```python
from build123d import *

# Parameters (mm, degrees)
ESTRUSIONE1_DEPTH                                    = 200
M10_LAMATURA_PER_VITE_A_COPERTURA_CILIND_D           = 11
M10_LAMATURA_PER_VITE_A_COPERTURA_CILIND_CBORE_D     = 18
M10_LAMATURA_PER_VITE_A_COPERTURA_CILIND_CBORE_DEPTH = 10
RIPETIZIONE_A_L1_COUNT                               = 5
RIPETIZIONE_A_L1_PITCH                               = 42
RIPETIZIONE_A_L1_COUNT_DIR2                          = 2
RIPETIZIONE_A_L1_PITCH_DIR2                          = 160
SMUSSO1_SIZE                                         = 3
ESTRUSIONE2_DEPTH                                    = 223.712819568
M10_TAPPED_HOLE1_D                                   = 8.5
M10_TAPPED_HOLE1_DEPTH                               = 17.5
M10_TAPPED_HOLE1_TIP                                 = 2.553657631
SCHIZZO10_R                                          = 4
ESTRUSIONE3_DEPTH                                    = 12
ESTRUSIONE5_DEPTH                                    = 200
SMUSSO2_SIZE                                         = 2


with BuildPart() as part:
    # Schizzo1 → Estrusione1 (new body)
    with BuildSketch(Plane(origin=(0, 0, 0), x_dir=(1, 0, 0), z_dir=(0, 1, 0))):
        Polygon((0, -95), (0, 95), (-24, 95), (-24, 90), (-19, 90), (-19, 70), (-24, 70), (-24, -70), (-19, -70), (-19, -90), (-24, -90), (-24, -95), align=None)
    extrude(amount=ESTRUSIONE1_DEPTH)

    # M10 Lamatura per vite a copertura cilind (through all)
    with Locations(Plane(origin=(0, 0, 0), x_dir=(0, 0, -1), z_dir=(1, 0, 0))):
        with Locations((-80, 184)):
            m10_lamatura_per_vite_a_copertura_cilind = CounterBoreHole(M10_LAMATURA_PER_VITE_A_COPERTURA_CILIND_D / 2, M10_LAMATURA_PER_VITE_A_COPERTURA_CILIND_CBORE_D / 2, M10_LAMATURA_PER_VITE_A_COPERTURA_CILIND_CBORE_DEPTH)

    # Ripetizione a L1: M10 Lamatura per vite a copertura cilind 5 × 2
    with Locations(*[(0, -i * RIPETIZIONE_A_L1_PITCH, -j * RIPETIZIONE_A_L1_PITCH_DIR2) for i in range(RIPETIZIONE_A_L1_COUNT) for j in range(RIPETIZIONE_A_L1_COUNT_DIR2) if (i, j) != (0, 0)]):
        add(m10_lamatura_per_vite_a_copertura_cilind, mode=Mode.SUBTRACT)

    # Smusso1
    smusso1_edges = [part.edges().sort_by_distance(p)[0] for p in [
        (0, 100, -95),
        (0, 100, 95),
    ]]
    chamfer(smusso1_edges, length=SMUSSO1_SIZE)

    # Schizzo4 → Estrusione2 (cut, through all)
    with BuildSketch(Plane(origin=(0, 200, 0), x_dir=(1, 0, 0), z_dir=(0, 1, 0))):
        Polygon((-22, -29.5), (-22, 29.5), (-31.824658815, 29.5), (-31.824658815, 0), (-31.824658815, -29.5), align=None)
    extrude(amount=-ESTRUSIONE2_DEPTH, mode=Mode.SUBTRACT)

    # M10 Tapped Hole1
    with Locations(Plane(origin=(0, 0, 0), x_dir=(0, 0, -1), z_dir=(1, 0, 0))):
        with Locations((-44, 169), (44, 169), (44, 31), (-44, 31)):
            Hole(M10_TAPPED_HOLE1_D / 2, depth=M10_TAPPED_HOLE1_DEPTH)
            with Locations((0, 0, -(M10_TAPPED_HOLE1_DEPTH + M10_TAPPED_HOLE1_TIP / 2))):  # 118° drill point
                Cone(0, M10_TAPPED_HOLE1_D / 2, M10_TAPPED_HOLE1_TIP, mode=Mode.SUBTRACT)

    # Schizzo10 → Estrusione3 (cut)
    with BuildSketch(Plane(origin=(0, 0, 0), x_dir=(0, 0, -1), z_dir=(1, 0, 0))):
        with Locations((0, 169)):
            Circle(SCHIZZO10_R)
        with Locations(Location((0, 31, 0), (0, 0, 180))):
            Circle(SCHIZZO10_R)
    extrude(amount=-ESTRUSIONE3_DEPTH, mode=Mode.SUBTRACT)

    # Schizzo12 → Estrusione5 (add)
    with BuildSketch(Plane(origin=(0, 200, 0), x_dir=(1, 0, 0), z_dir=(0, 1, 0))):
        Polygon((-24, 29.5), (-40, 24.5), (-40, -24.5), (-24, -29.5), (-22, -29.5), (-22, 29.5), align=None)
    extrude(amount=-ESTRUSIONE5_DEPTH)

    # Smusso2
    smusso2_edges = [part.edges().sort_by_distance(p)[0] for p in [
        (-24, 200, 49.75),
        (-32, 200, -27),
        (-40, 200, 0),
        (-32, 200, 27),
        (-24, 200, -49.75),
    ]]
    chamfer(smusso2_edges, length=SMUSSO2_SIZE)


solid = part.part
```
Design review of the part built by this model. Coordinates are the model's own, in mm. A direction names the side the tool comes from. Coordinates: 2 decimals unless noted, no trailing zeros. Order: outer loops, then holes, each group sorted by start corner. A loop starts at its lowest first (then second) coordinate and runs counter-clockwise, first axis right, second up. Notation, with made-up numbers: (70.5, 32) - (113.5, 32) arc R18 ccw to (113.5, 41) - close; hole circle Ø8 at (-36.5, 66). An arc over 180 degrees is marked (long way). Answer in a Markdown table with one row per item.
(1) Consider section B-B on z = 0. State the section outline as (x, y) points.
Checked values:
| item | result |
|---|---|
| outline | (-40, 0) - (0, 0) - (0, 27) - (-12, 27) - (-12, 35) - (0, 35) - (0, 165) - (-12, 165) - (-12, 173) - (0, 173) - (0, 200) - (-38, 200) - (-40, 198) - close |
(2) The part is to be moulded in two halves that separate along Z. For faces 4 (the flat face through (-32, 100, 27)), 5 (the cylindrical face through (-4.93, 18.703, -88.584)), 6 (the flat face through (-10, 104, 76)), 7 (the flat face through (0, 99, 1)), say which applies: released by +Z, released by -Z, zero draft, split by the parting line, or undercut.
Checked values:
| item | result |
|---|---|
| face 4 | released by +Z |
| face 5 | undercut |
| face 6 | undercut |
| face 7 | zero draft |
(3) Wall thickness on line 1 along Y through (x, z) = (-16, 80); line 2 along Z through (x, y) = (-5, 31); line 3 along Y through (x, z) = (-6, 80): over which ranges is each line inside the solid? List them lowest first. Write a range as from..to.
Checked values:
| item | result |
|---|---|
| line 1 | 0..10.5, 21.5..52.5, 63.5..94.5, 105.5..136.5, 147.5..178.5, 189.5..200 |
| line 2 | -95..-48.25, -39.75..-4, 4..39.75, 48.25..95 |
| line 3 | 0..7, 25..49, 67..91, 109..133, 151..175, 193..200 |
(4) Consider section D-D on z = -64. State the section outline as (x, y) points, plus the area to 3 significant figures.
Checked values:
| item | result |
|---|---|
| outline | (-24, 0) - (0, 0) - (0, 200) - (-22, 200) - (-24, 198) - close |
| area | 4,800 mm^2 |
(5) Clearance check with flat-ended pins moving along their axes: pin 1 (6 mm diameter, centred on x = -34, y = 170, fed in from +Z); pin 2 (14.5 mm diameter, centred on y = 58, z = 80, fed in from +X); pin 3 (10 mm diameter, centred on y = 100, z = 80, fed in from +X); pin 4 (17.5 mm diameter, centred on y = 58, z = 80, fed in from -X). State where each tip first meets the part, or that it passes through.
Checked values:
| item | result |
|---|---|
| pin 1 | z = 27.31 |
| pin 2 | x = -10 |
| pin 3 | through |
| pin 4 | x = -19 |
(6) For faces 1 (the cylindrical face through (-14.563, 16.242, 74.505)), 2 (the flat face through (-19, 99, -73)), 3 (the flat face through (-10, 104, -84)), list the 3-axis set-ups (+Z, -Z, +X, -X, +Y, -Y) from which the entire face can be reached by the end or side of a thin tool; tool diameter is ignored.
Checked values:
| item | result |
|---|---|
| face 1 | +X, -X |
| face 2 | -X, +Y, -Y |
| face 3 | +X |
(7) Consider section A-A on y = 100. Give the number of separate pieces and of enclosed holes in the cut face, plus the area to 3 significant figures.
Checked values:
| item | result |
|---|---|
| separate pieces | 3 |
| enclosed holes | 0 |
| area | 4,660 mm^2 |
